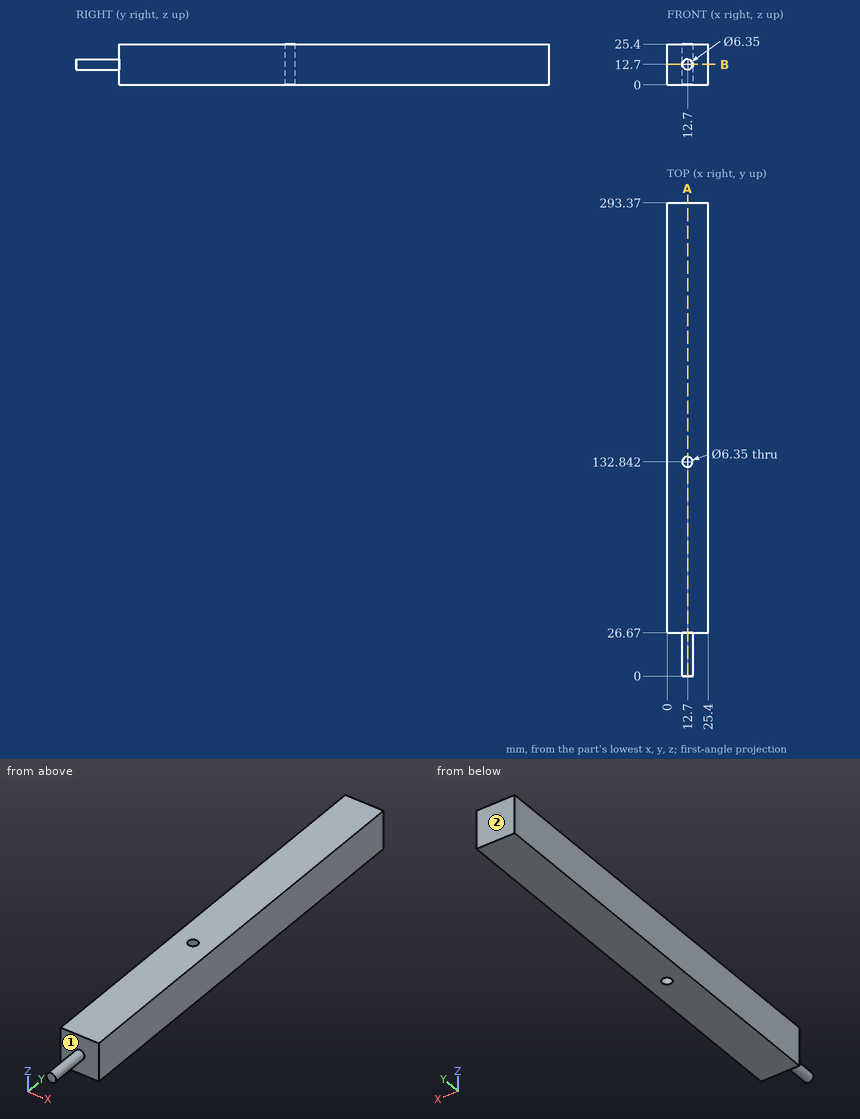
Check sheet for the drawn part. Datum: minimum x, y, z corner. Units: mm. A direction names the side the tool comes from. Coordinates: 2 decimals unless noted, no trailing zeros. Loops run counter-clockwise (first coordinate to the right, second up) from the corner with the lowest first, then second, coordinate; pieces in that order, holes last. Notation, with made-up numbers: (86, -33) -> (116, -33) arc R16 cw to (116, -15) -> close; hole circle Ø1 at (43, 58.5). An arc over 180 degrees is marked (long way). Answer as a JSON object with one key per item and string values. Group by question number.
Item 1: Depth check by flat-ended pin: pin 1 (12.5 mm diameter, centred on x = 10, z = 8.5, fed in from -Y); pin 2 (8 mm diameter, centred on x = 17.5, z = 4.5, fed in from -Y). Enter the tip coordinate at first touch or a pass-through.
Item 2: Sectioned sample at B-B on z = 12.7. Record the boundary of the cut face in (x, y) (3 decimals), plus the area to 3 significant figures.
Item 3: Scan lines: probe 1 along Y at (x, z) = (12.7, 18.5); probe 2 along Y at (x, z) = (12.7, 15.5); probe 3 along Y at (x, z) = (21, 21.5). Record each from-to range of solid material in increasing order.
Item 4: Sectioned sample at A-A on x = 12.7. Record the boundary of the cut face in (y, z) (3 decimals), plus the area to 3 significant figures.
Item 5: Tool access check on the marked faces 1 and 2. Record the directions out of +Z, -Z, +X, -X, +Y, -Y that give a thin tool (end or side, any length) a straight path to the whole face; none if there is none.
Evaluation:
{
 "1": {"pin 1": "stops at y = 0", "pin 2": "stops at y = 26.67"},
 "2": {"outline": "(0, 26.67) -> (9.525, 26.67) -> (9.525, 0) -> (15.875, 0) -> (15.875, 26.67) -> (25.4, 26.67) -> (25.4, 293.37) -> (0, 293.37) -> close; hole circle Ø6.35 at (12.7, 132.842)", "area": "6,910 mm²"},
 "3": {"probe 1": "y = 26.67 to 129.67, 136.02 to 293.37", "probe 2": "y = 0 to 129.67, 136.02 to 293.37", "probe 3": "y = 26.67 to 293.37"},
 "4": {"outline": "(0, 9.525) -> (26.67, 9.525) -> (26.67, 0) -> (129.667, 0) -> (129.667, 25.4) -> (26.67, 25.4) -> (26.67, 15.875) -> (0, 15.875) -> close; (136.017, 0) -> (293.37, 0) -> (293.37, 25.4) -> (136.017, 25.4) -> close", "area": "6,780 mm²"},
 "5": {"face 1": "-Y", "face 2": "+Z, -Z, +X, -X, +Y"}
}
